Input: part model. Units: mm. Frame: model coordinates. A direction names the side the tool comes from. Round coordinates to 2 decimals unless told otherwise and drop trailing zeros. Order: outer loops, then holes, each group sorted by start corner. A loop starts at its lowest first (then second) coordinate and runs counter-clockwise, first axis right, second up. Notation, with made-up numbers: (45.5, 29) -> (62.5, 29) arc R30 ccw to (62.5, 51) -> close; hole circle Ø4 at (77, 67). An arc over 180 degrees is marked (long way). Use a Markdown table: item, result.
from build123d import *

# Parameters (mm, degrees)
LOFT3_START         = -2.5
LOFT3_DEPTH         = 5
SKETCH7_W           = 4
SKETCH7_H           = 5
BOSS_EXTRUDE1_DEPTH = 5


# Read off the part's stored shape, not the designer's step: Loft3
with BuildPart() as part:
    # Loft3 outline → Loft3 (new body)
    with BuildSketch(Plane.XY.offset(LOFT3_START)):
        Polygon((5.008763306, -99.9), (9.508763306, -99.9), (9.508763306, 0), (3.508763306, 0), align=None)
    extrude(amount=LOFT3_DEPTH)

    # Sketch7 → Boss-Extrude1 (add)
    with BuildSketch(Plane.XY.offset(2.5)):
        with Locations((11.508763306, -2.5)):
            Rectangle(SKETCH7_W, SKETCH7_H)
    extrude(amount=-BOSS_EXTRUDE1_DEPTH)


solid = part.part
1) Contact query for flat-ended pins moving along their axis: P1, Ø1, axis at y = -47, z = -0.5, coming from the -X side; P2, Ø2.5, axis at y = -72.5, z = -1, coming from the +X side. Output: stop coordinate, or through.
Answer key:
| item | result |
|---|---|
| P1 | stops at x = 4.21 |
| P2 | stops at x = 9.51 |
2) Ray query, probe 1 along Y at (x, z) = (9.75, 2); probe 2 along X at (y, z) = (-79, -0.15); probe 3 along X at (y, z) = (-29, 0.9). Return the intervals inside material, ascending.
Answer key:
| item | result |
|---|---|
| probe 1 | y = -5 to 0 |
| probe 2 | x = 4.69 to 9.51 |
| probe 3 | x = 3.94 to 9.51 |
3) Cut plane A-A on z = -0.35. Return loops of the section in (x, y), and give its area (3 significant figures).
Answer key:
| item | result |
|---|---|
| outline | (3.51, 0) -> (5.01, -99.9) -> (9.51, -99.9) -> (9.51, -5) -> (13.51, -5) -> (13.51, 0) -> close |
| area | 544 mm^2 |
4) Set-up query: faces 1 (the face through (7, -38, 2.5)), 2 (the face through (11, -5, 0)). Return all of +Z, -Z, +X, -X, +Y, -Y with unobstructed straight access to the full face (end or side cutting, diameter ignored); none if empty.
Answer key:
| item | result |
|---|---|
| face 1 | +Z, +X, -X, +Y, -Y |
| face 2 | +Z, -Z, +X, -Y |
5) Cut plane C-C on y = -6.5. Return loops of the section in (x, z).
Answer key:
| item | result |
|---|---|
| outline | (3.61, -2.5) -> (9.51, -2.5) -> (9.51, 2.5) -> (3.61, 2.5) -> close |
6) Cut plane B-B on x = 11. Return loops of the section in (y, z).
Answer key:
| item | result |
|---|---|
| outline | (-5, -2.5) -> (0, -2.5) -> (0, 2.5) -> (-5, 2.5) -> close |
